```python
from build123d import *

# Parameters (mm, degrees)
SKETCH1_R           = 6.35
SKETCH1_R_2         = 3.175
BOSS_EXTRUDE1_DEPTH = 4.7625
SKETCH1_3_R         = 7.14375
SKETCH1_3_R_2       = 6.35
BOSS_EXTRUDE2_DEPTH = 1.2065
FILLET1_R           = 0.254


with BuildPart() as part:
    # Sketch1 → Boss-Extrude1 (new body)
    with BuildSketch(Plane(origin=(0, 0, 0), x_dir=(1, 0, 0), z_dir=(0, 1, 0))):
        Circle(SKETCH1_R)
        Circle(SKETCH1_R_2, mode=Mode.SUBTRACT)
    extrude(amount=BOSS_EXTRUDE1_DEPTH)

    # Sketch1<3> → Boss-Extrude2 (add)
    with BuildSketch(Plane(origin=(0, 0, 0), x_dir=(1, 0, 0), z_dir=(0, 1, 0))):
        Circle(SKETCH1_3_R)
        Circle(SKETCH1_3_R_2, mode=Mode.SUBTRACT)
    extrude(amount=BOSS_EXTRUDE2_DEPTH)

    # Fillet1
    fillet1_edges = [part.edges().sort_by_distance(p)[0] for p in [
        (-7.14375, 1.2065, 0),
        (-6.35, 4.7625, 0),
        (-7.14375, 0, 0),
    ]]
    fillet(fillet1_edges, radius=FILLET1_R)


solid = part.part
```
The model under review builds one solid part; all positions refer to its coordinate system, in mm. A direction names the side the tool comes from. Round coordinates to 2 decimals unless told otherwise and drop trailing zeros. Write each loop counter-clockwise with the first axis right and the second up, starting at its lowest first coordinate (ties: lowest second). Pieces come first, ordered by that corner, then holes. Notation, with made-up numbers: M 68,84 L 118,84 A16 cw 118,94 Z; hole C -26,61.25 d9. An arc over 180 degrees is marked long. Use CSV: the item, a comma, the result in double quotes. Start each with the question number.
(1) The part is to be moulded in two halves that separate along Z. For faces 1 (the face through (3, 0, -2)), 2 (the face through (-0.69, 2.35, 3.1)), 3 (the face through (-1.38, 2.83, 6.2)), say which applies: +Z half, -Z half, draft (parallel to the pull), parting line (faces both ways), or undercut.
(2) We need section C-C, the plane y = 3.95. State the section outline as (x, z) points (3 decimals), then the cut area to 3 significant figures.
(3) For line 1 along Z through (x, y) = (0, 2.15) (3 decimals); line 2 along X through (y, z) = (1, 0) (3 decimals), list the stretches that pass through material, from the lowest coordinate up.
(4) Tool access review of faces 4 (the face through (3, 1.206, 6)), 5 (the face through (3, 4.762, 3)): name each direction out of +Z, -Z, +X, -X, +Y, -Y from which nothing blocks a thin tool from reaching the whole face with its end or side.
Findings:
1,face 1,"draft"
1,face 2,"undercut"
1,face 3,"parting line"
2,outline,"C 0,0 d12.7; hole C 0,0 d6.35"
2,area,"95.0 mm^2"
3,line 1,"-6.35 to -3.175, 3.175 to 6.35"
3,line 2,"-7.139 to -3.175, 3.175 to 7.139"
4,face 4,"+Y"
4,face 5,"+Z, -Z, +X, -X, +Y"
